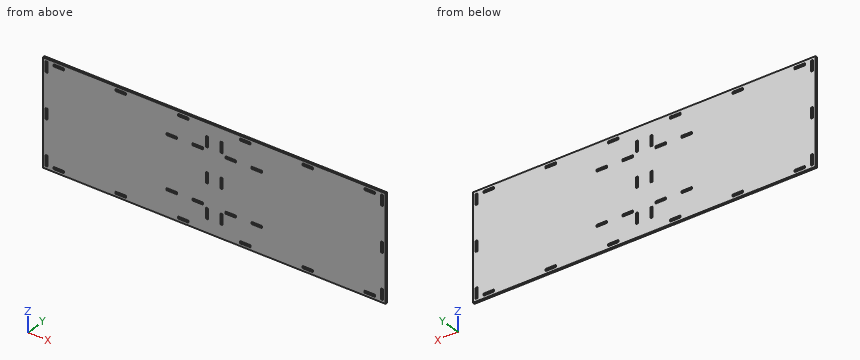
```python
from build123d import *

# Parameters (mm, degrees)
SKETCH1_W           = 660
SKETCH1_H           = 200
SKETCH1_W_2         = 20
SKETCH1_H_2         = 4
SKETCH1_W_3         = 4
SKETCH1_H_3         = 20
BOSS_EXTRUDE1_DEPTH = 4


with BuildPart() as part:
    # Sketch1 → Boss-Extrude1 (new body)
    with BuildSketch(Plane(origin=(0, 0, 0), x_dir=(1, 0, 0), z_dir=(0, 1, 0))):
        Rectangle(SKETCH1_W, SKETCH1_H)
        with Locations((-82, 49.859697176)):
            Rectangle(SKETCH1_W_2, SKETCH1_H_2, mode=Mode.SUBTRACT)
        with Locations((-32, 49.859697176)):
            Rectangle(SKETCH1_W_2, SKETCH1_H_2, mode=Mode.SUBTRACT)
        with Locations((-82, -50.140302824)):
            Rectangle(SKETCH1_W_2, SKETCH1_H_2, mode=Mode.SUBTRACT)
        with Locations((-32, -50.140302824)):
            Rectangle(SKETCH1_W_2, SKETCH1_H_2, mode=Mode.SUBTRACT)
        with Locations((-14, 64.859697176)):
            Rectangle(SKETCH1_W_3, SKETCH1_H_3, mode=Mode.SUBTRACT)
        with Locations((14, 64.859697176)):
            Rectangle(SKETCH1_W_3, SKETCH1_H_3, mode=Mode.SUBTRACT)
        with Locations((32, 49.859697176)):
            Rectangle(SKETCH1_W_2, SKETCH1_H_2, mode=Mode.SUBTRACT)
        with Locations((82, 49.859697176)):
            Rectangle(SKETCH1_W_2, SKETCH1_H_2, mode=Mode.SUBTRACT)
        with Locations((-14, 0)):
            Rectangle(SKETCH1_W_3, SKETCH1_H_3, mode=Mode.SUBTRACT)
        with Locations((14, -0.140302824)):
            Rectangle(SKETCH1_W_3, SKETCH1_H_3, mode=Mode.SUBTRACT)
        with Locations((32, -50.140302824)):
            Rectangle(SKETCH1_W_2, SKETCH1_H_2, mode=Mode.SUBTRACT)
        with Locations((14, -65.140302824)):
            Rectangle(SKETCH1_W_3, SKETCH1_H_3, mode=Mode.SUBTRACT)
        with Locations((82, -50.140302824)):
            Rectangle(SKETCH1_W_2, SKETCH1_H_2, mode=Mode.SUBTRACT)
        with Locations((-323, -85)):
            Rectangle(SKETCH1_W_3, SKETCH1_H_3, mode=Mode.SUBTRACT)
        with Locations((-323, 85)):
            Rectangle(SKETCH1_W_3, SKETCH1_H_3, mode=Mode.SUBTRACT)
        with Locations((323, -85)):
            Rectangle(SKETCH1_W_3, SKETCH1_H_3, mode=Mode.SUBTRACT)
        with Locations((-323, 0)):
            Rectangle(SKETCH1_W_3, SKETCH1_H_3, mode=Mode.SUBTRACT)
        with Locations((323, 0)):
            Rectangle(SKETCH1_W_3, SKETCH1_H_3, mode=Mode.SUBTRACT)
        with Locations((323, 85)):
            Rectangle(SKETCH1_W_3, SKETCH1_H_3, mode=Mode.SUBTRACT)
        with Locations((-300, 93)):
            Rectangle(SKETCH1_W_2, SKETCH1_H_2, mode=Mode.SUBTRACT)
        with Locations((-180, 93)):
            Rectangle(SKETCH1_W_2, SKETCH1_H_2, mode=Mode.SUBTRACT)
        with Locations((-60, 93)):
            Rectangle(SKETCH1_W_2, SKETCH1_H_2, mode=Mode.SUBTRACT)
        with Locations((300, 93)):
            Rectangle(SKETCH1_W_2, SKETCH1_H_2, mode=Mode.SUBTRACT)
        with Locations((-14, -65.140302824)):
            Rectangle(SKETCH1_W_3, SKETCH1_H_3, mode=Mode.SUBTRACT)
        with Locations((180, 93)):
            Rectangle(SKETCH1_W_2, SKETCH1_H_2, mode=Mode.SUBTRACT)
        with Locations((60, 93)):
            Rectangle(SKETCH1_W_2, SKETCH1_H_2, mode=Mode.SUBTRACT)
        with Locations((300, -93)):
            Rectangle(SKETCH1_W_2, SKETCH1_H_2, mode=Mode.SUBTRACT)
        with Locations((180, -93)):
            Rectangle(SKETCH1_W_2, SKETCH1_H_2, mode=Mode.SUBTRACT)
        with Locations((60, -93)):
            Rectangle(SKETCH1_W_2, SKETCH1_H_2, mode=Mode.SUBTRACT)
        with Locations((-60, -93)):
            Rectangle(SKETCH1_W_2, SKETCH1_H_2, mode=Mode.SUBTRACT)
        with Locations((-180, -93)):
            Rectangle(SKETCH1_W_2, SKETCH1_H_2, mode=Mode.SUBTRACT)
        with Locations((-300, -93)):
            Rectangle(SKETCH1_W_2, SKETCH1_H_2, mode=Mode.SUBTRACT)
    extrude(amount=BOSS_EXTRUDE1_DEPTH)


solid = part.part
```
Source: CAD feature listing. Evaluate the final solid. Frame: model axes, mm. Coordinates: 2 decimals unless noted, no trailing zeros. Loops run counter-clockwise (first coordinate to the right, second up) from the corner with the lowest first, then second, coordinate; pieces in that order, holes last. Notation, with made-up numbers: (16, 67.5) - (37, 67.5) arc R22 ccw to (37, 80.5) - close; hole circle Ø2 at (-22, -22). An arc over 180 degrees is marked (long way). Answer as CSV lines item,"result".
1. Section B-B (y = 3.3). Count the separate pieces of the cut face and the enclosed holes in it, then the cut area to 3 significant figures.
Established:
separate pieces,"1"
enclosed holes,"32"
area,"129,000 mm2"
2. Contact query for a flat-ended pin moving along its axis: pin 1 (6 mm diameter, centred on x = -183.5, z = -52, fed in from -Y). Output: stop coordinate, or through.
Established:
pin 1,"stops at y = 0"
3. Ray query, line 1 (X direction, y = 0.45, z = 82.5); line 2 (X direction, y = 2.4, z = -73); line 3 (Z direction, x = 80.5, y = 0.3). Return the intervals inside material, ascending.
Established:
line 1,"x = -330 to -325, -321 to 321, 325 to 330"
line 2,"x = -330 to -16, -12 to 12, 16 to 330"
line 3,"z = -100 to -51.86, -47.86 to 48.14, 52.14 to 100"
4. Section A-A (x = 31). Return loops of the section in (y, z), then the cut area to 3 significant figures.
Established:
outline,"(0, -100) - (4, -100) - (4, -51.86) - (0, -51.86) - close; (0, -47.86) - (4, -47.86) - (4, 48.14) - (0, 48.14) - close; (0, 52.14) - (4, 52.14) - (4, 100) - (0, 100) - close"
area,"768 mm2"
